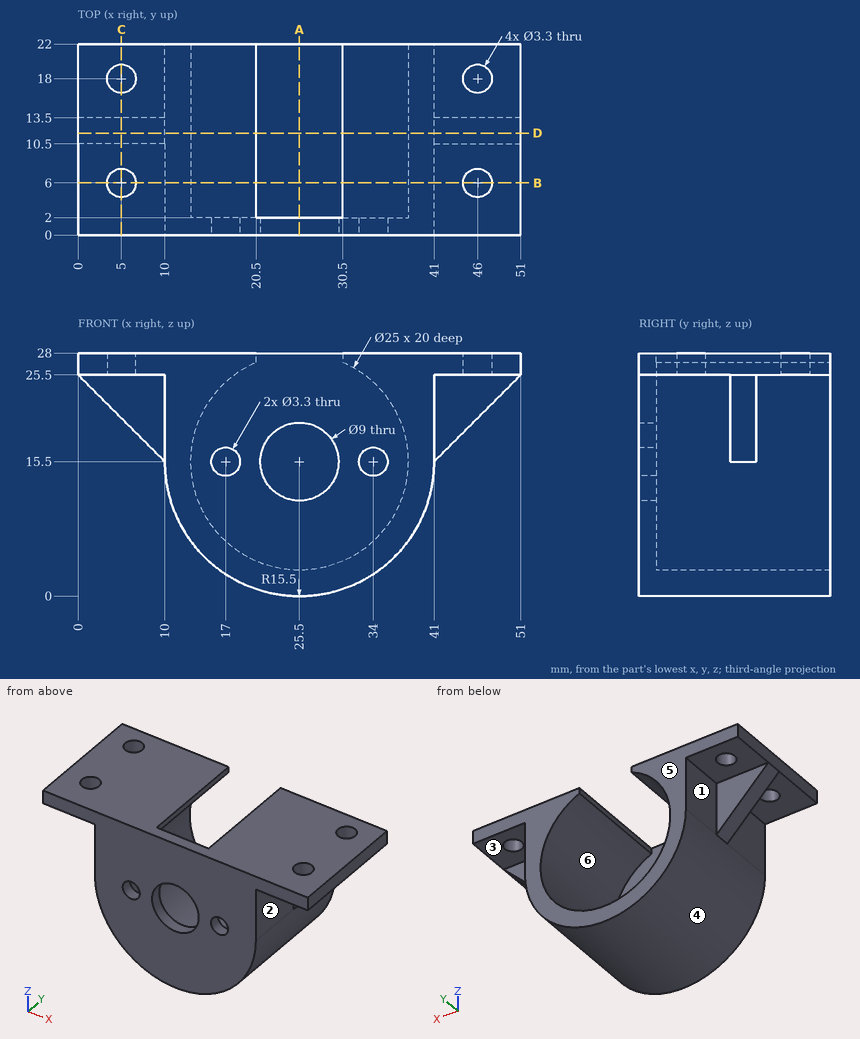
Input: dimensioned drawing with shaded views. Units: mm. Origin: part minimum x, y, z. A direction names the side the tool comes from. Round coordinates to 2 decimals unless told otherwise and drop trailing zeros. Write each loop counter-clockwise with the first axis right and the second up, starting at its lowest first coordinate (ties: lowest second). Pieces come first, ordered by that corner, then holes. Notation, with made-up numbers: (68.5, -31) - (104.5, -31) arc R7 ccw to (104.5, -19) - close; hole circle Ø4 at (14.5, 8). An arc over 180 degrees is marked (long way). Write item = value, one per line.
(1) Section query B-B on y = 6. Output: boundary loops of the cut face in (x, z).
Geometry check:
outline = (0, 25.5) - (3.35, 25.5) - (3.35, 28) - (0, 28) - close; (6.65, 25.5) - (10, 25.5) - (10, 15.5) arc R15.5 ccw to (41, 15.5) - (41, 25.5) - (44.35, 25.5) - (44.35, 28) - (30.5, 28) - (30.5, 26.96) arc R12.5 cw (long way) to (20.5, 26.96) - (20.5, 28) - (6.65, 28) - close; (47.65, 25.5) - (51, 25.5) - (51, 28) - (47.65, 28) - close
(2) Section query D-D on y = 11.75. Output: boundary loops of the cut face in (x, z).
Geometry check:
outline = (0, 25.5) - (10, 15.5) arc R15.5 ccw to (41, 15.5) - (51, 25.5) - (51, 28) - (30.5, 28) - (30.5, 26.96) arc R12.5 cw (long way) to (20.5, 26.96) - (20.5, 28) - (0, 28) - close
(3) Contact query for flat-ended pins moving along their axis: pin 1 Ø7 at (x, z) = (25.5, 15.5) entering from -Y; pin 2 Ø7 at (x, y) = (47.5, 20) entering from -Z; pin 3 Ø9.5 at (y, z) = (19.5, 19.5) entering from -X; pin 4 Ø1.5 at (y, z) = (15.5, 12) entering from -X. Output: stop coordinate, or through.
Geometry check:
pin_1 = through
pin_2 = 25.5
pin_3 = 10
pin_4 = 10.25
(4) Pull-direction query (X, two-part tool) for the marked faces 4, 5 and 6; classes: +X half, -X half, draft (parallel to the pull), parting line (faces both ways), or undercut.
Geometry check:
face_4 = parting line
face_5 = draft
face_6 = undercut
(5) Section query C-C on x = 5. Output: boundary loops of the cut face in (y, z), then the cut area to 3 significant figures.
Geometry check:
outline = (0, 25.5) - (4.35, 25.5) - (4.35, 28) - (0, 28) - close; (7.65, 25.5) - (10.5, 25.5) - (10.5, 20.5) - (13.5, 20.5) - (13.5, 25.5) - (16.35, 25.5) - (16.35, 28) - (7.65, 28) - close; (19.65, 25.5) - (22, 25.5) - (22, 28) - (19.65, 28) - close
area = 53.5 mm^2
(6) Section query A-A on x = 25.5. Output: boundary loops of the cut face in (y, z).
Geometry check:
outline = (0, 0) - (22, 0) - (22, 3) - (2, 3) - (2, 11) - (0, 11) - close; (0, 20) - (2, 20) - (2, 28) - (0, 28) - close
(7) Access query for the marked faces 1, 2 and 3. Directions: +Z, -Z, +X, -X, +Y, -Y. A direction counts if a zero-diameter tool reaches every point of the face in a straight line with its end or side. Return the directions, or none.
Geometry check:
face_1 = -Z, -X, +Y
face_2 = -Z, +X, -Y
face_3 = -Z, +X, +Y
(8) Material intervals for probe 1 along X at (y, z) = (0.8, 15.5); probe 2 along Y at (x, z) = (46, 26.3); probe 3 along X at (y, z) = (14, 15.5), sorted ascending.
Geometry check:
probe_1 = 10 to 15.35, 18.65 to 21, 30 to 32.35, 35.65 to 41
probe_2 = 0 to 4.35, 7.65 to 16.35, 19.65 to 22
probe_3 = 10 to 13, 38 to 41
